from build123d import *

# Parameters (mm, degrees)
EXTRUDE_1_DEPTH        = 570
HOLE_WIZARD_M6_1_D     = 5
HOLE_WIZARD_M6_1_DEPTH = 17
HOLE_WIZARD_M6_1_TIP   = 1.502151548
HOLE_WIZARD_M6_2_D     = 5
HOLE_WIZARD_M6_2_DEPTH = 17
HOLE_WIZARD_M6_2_TIP   = 1.502151548


with BuildPart() as part:
    # 草图1 → 凸台-拉伸1 (new body)
    with BuildSketch(Plane.XY):
        Polygon((10, 0.25), (10, -0.25), (12, -2.25), (12, -3), (10, -5), (10, -10), (30, -10), (30, 10), (10, 10), (10, 5), (12, 3), (12, 2.25), align=None)
    extrude_1 = extrude(amount=-EXTRUDE_1_DEPTH)

    # 镜向1: 凸台-拉伸1 across plane
    add(extrude_1.mirror(Plane(origin=(30, 0, 0), x_dir=(0, 0, 1), z_dir=(1, 0, 0))))

    # M6 螺纹孔1
    with Locations(Plane(origin=(0, 0, -570), x_dir=(-1, 0, 0), z_dir=(0, 0, -1))):
        with Locations((-40, 0), (-20, 0)):
            Hole(HOLE_WIZARD_M6_1_D / 2, depth=HOLE_WIZARD_M6_1_DEPTH)
            with Locations((0, 0, -(HOLE_WIZARD_M6_1_DEPTH + HOLE_WIZARD_M6_1_TIP / 2))):  # 118° drill point
                Cone(0, HOLE_WIZARD_M6_1_D / 2, HOLE_WIZARD_M6_1_TIP, mode=Mode.SUBTRACT)

    # M6 螺纹孔2
    with Locations(Plane.XY):
        with Locations((19.572746266, 0), (40.572746266, 0)):
            Hole(HOLE_WIZARD_M6_2_D / 2, depth=HOLE_WIZARD_M6_2_DEPTH)
            with Locations((0, 0, -(HOLE_WIZARD_M6_2_DEPTH + HOLE_WIZARD_M6_2_TIP / 2))):  # 118° drill point
                Cone(0, HOLE_WIZARD_M6_2_D / 2, HOLE_WIZARD_M6_2_TIP, mode=Mode.SUBTRACT)


solid = part.part
Design review of the part built by this model. Coordinates are the model's own, in mm. Coordinates: 2 decimals unless noted, no trailing zeros. Order: outer loops, then holes, each group sorted by start corner. A loop starts at its lowest first (then second) coordinate and runs counter-clockwise, first axis right, second up. Notation, with made-up numbers: (37.5, 86.5) - (42.5, 86.5) arc R20 ccw to (42.5, 91.5) - close; hole circle Ø1 at (17, -34.5). An arc over 180 degrees is marked (long way). Put each result on its own line as item: value.
1) Insertion check: P1, Ø8, axis at x = 40.57, y = 0, coming from the -Z side; P2, Ø0.6, axis at y = -2.5, z = -278.5, coming from the -X side; P3, Ø1.5, axis at y = 3.5, z = -221, coming from the -X side; P4, Ø0.8, axis at y = 2.5, z = -381.5, coming from the +X side. Each pin has a flat end and moves straight along its axis. Give the tip position at first contact, or say it passes through.
Response values:
P1: stops at z = -570
P2: stops at x = 11.95
P3: stops at x = 10.75
P4: stops at x = 48.15
2) Wall thickness on L1, parallel to X at y = 0, z = -11.75; L2, parallel to Y at x = 40, z = -559.5; L3, parallel to X at y = 2.5, z = -379.5: over which ranges is each line inside the solid? List them lowest first. Write a range as from..to.
Response values:
L1: x = 10..17.07, 22.07..38.07, 43.07..50
L2: y = -10..-2.5, 2.5..10
L3: x = 12..48
3) Take a section at A-A, the plane z = -490. Give the boundary of the cut face in (x, y), and give its area (3 significant figures).
Response values:
outline: (10, -10) - (50, -10) - (50, -5) - (48, -3) - (48, -2.25) - (50, -0.25) - (50, 0.25) - (48, 2.25) - (48, 3) - (50, 5) - (50, 10) - (10, 10) - (10, 5) - (12, 3) - (12, 2.25) - (10, 0.25) - (10, -0.25) - (12, -2.25) - (12, -3) - (10, -5) - close
area: 778 mm²
